```python
from build123d import *

# Parameters (mm, degrees)
SKETCH1_W           = 119.38
SKETCH1_H           = 78.74
BOSS_EXTRUDE1_DEPTH = 22.86
SKETCH2_W           = 12
SKETCH2_H           = 4.5
CUT_EXTRUDE1_DEPTH  = 2.54
SKETCH3_R           = 5.06527112
SKETCH3_R_2         = 3.320502589
SKETCH3_R_3         = 2.836896815
CUT_EXTRUDE2_DEPTH  = 2.54


with BuildPart() as part:
    # Sketch1 → Boss-Extrude1 (new body)
    with BuildSketch(Plane(origin=(0, 0, 0), x_dir=(1, 0, 0), z_dir=(0, 1, 0))):
        with Locations((59.69, 39.37)):
            Rectangle(SKETCH1_W, SKETCH1_H)
    extrude(amount=BOSS_EXTRUDE1_DEPTH)

    # Sketch2 → Cut-Extrude1 (cut)
    with BuildSketch(Plane(origin=(119.38, 0, 0), x_dir=(0, 0, -1), z_dir=(1, 0, 0))):
        with Locations((35.78, 11.72)):
            Rectangle(SKETCH2_W, SKETCH2_H)
        with Locations((13.62, 11.72)):
            Rectangle(SKETCH2_W, SKETCH2_H)
    extrude(amount=-CUT_EXTRUDE1_DEPTH, mode=Mode.SUBTRACT)

    # Sketch3 → Cut-Extrude2 (cut)
    with BuildSketch(Plane(origin=(0, 22.86, 0), x_dir=(1, 0, 0), z_dir=(0, 1, 0))):
        with Locations((94.579217674, 39.37)):
            Circle(SKETCH3_R)
        with Locations((94.579217674, 54.530950953)):
            Circle(SKETCH3_R_2)
        with Locations((94.579217674, 63.919322254)):
            Circle(SKETCH3_R_3)
        with Locations((94.579217674, 25.985227401)):
            Circle(SKETCH3_R_3)
        with Locations((94.579217674, 15.074417511)):
            Circle(SKETCH3_R_3)
    extrude(amount=-CUT_EXTRUDE2_DEPTH, mode=Mode.SUBTRACT)


solid = part.part
```
Could you check a few things on this model? Use its own coordinates, in mm. A direction names the side the tool comes from. Round coordinates to 2 decimals unless told otherwise and drop trailing zeros. Put each result on its own line as item: value.
Q1. Please list where these lines run through material, in increasing order: line 1 (X direction, y = 21.75, z = -39.37); line 2 (X direction, y = 11, z = -31.5). Write a range as from..to.
Checks:
line 1: 0..89.51, 99.64..119.38
line 2: 0..116.84
Q2. For pin 1 Ø6 at (x, z) = (94.58, -39.37) entering from +Y, with a flat end and sliding along its axis, tell me the tip position at first contact or that it passes through.
Checks:
pin 1: y = 20.32
Q3. Which directions (+Z, -Z, +X, -X, +Y, -Y) give clear straight access to the entire face, cutting with the end or side of a thin tool? Please do faces 1 (the flat face through (95, 20.32, -55)), 2 (the flat face through (118, 9.47, -36)), 3 (the flat face through (0, 11, -39)).
Checks:
face 1: +Y
face 2: +X
face 3: +Z, -Z, -X, +Y, -Y
Q4. Thinking about a two-plate mould opening in Y: for faces 4 (the cylindrical face through (94.147, 21.608, -57.823)), 5 (the flat face through (95, 20.32, -26)), 6 (the flat face through (116.84, 12, -14)), which applies, pulls with the +Y half, pulls with the -Y half, needs draft (parallel to the pull), parting line crosses it, or undercut?
Checks:
face 4: needs draft
face 5: pulls with the +Y half
face 6: undercut
